from build123d import *
from build123d.topology import SkipClean

# Parameters (mm, degrees)
BOSS_EXTRUDE1_DEPTH     = 12
CUT_EXTRUDE1_DEPTH      = 35.61106579391691
CUT_EXTRUDE1_DEPTH_BACK = 35.61106579391691
BOSS_EXTRUDE2_DEPTH     = 8
CUT_EXTRUDE2_DEPTH      = 2.5
CUT_EXTRUDE3_DEPTH      = 5
SKETCH8_R               = 1.4999999999999996
BOSS_EXTRUDE3_DEPTH     = 5.499999999999998
CUT_EXTRUDE4_DEPTH      = 35.61106579391691
CUT_EXTRUDE4_DEPTH_BACK = 35.61106579391691
SKETCH9_W               = 12
SKETCH9_H               = 6.50766833090351
CUT_EXTRUDE5_DEPTH      = 1


with BuildPart() as part:
    # Sketch1 → Boss-Extrude1 (new body)
    with BuildSketch(Plane.XY):
        with BuildLine():
            Line((-56.57427779976257, 0), (-40.57427779976257, 0))
            Line((-40.57427779976257, 0), (-42.06660946885906, 24.955419174788705))
            ThreePointArc((-42.06660946885906, 24.955419174788705), (-48.57427779976256, 31.463087505692204), (-55.08194613066607, 24.955419174788705))
            Line((-55.08194613066607, 24.955419174788705), (-56.57427779976257, 0))
        make_face()
    extrude(amount=BOSS_EXTRUDE1_DEPTH)

    # Sketch3 → Cut-Extrude1 (cut, two sides: drawn at the far end of the back side and taken through both)
    with BuildSketch(Plane(origin=(-48.57427779976257, 0, 0), x_dir=(0, 0, -1), z_dir=(1, 0, 0)).offset(-CUT_EXTRUDE1_DEPTH_BACK)):
        Polygon((-12, 6.613954943904592), (-12, 0), (-4, -4.9e-16), align=None)
    extrude(amount=CUT_EXTRUDE1_DEPTH + CUT_EXTRUDE1_DEPTH_BACK, mode=Mode.SUBTRACT)

    # Sketch6 → Boss-Extrude2 (add, symmetric)
    with BuildSketch(Plane(origin=(-48.57427779976257, 0, 0), x_dir=(0, 0, -1), z_dir=(1, 0, 0))):
        with BuildLine():
            ThreePointArc((-2.9999999999999982, -1.1000000000000008), (-3.0526985696936526, -0.5401658469562882), (-3.2089428526094457, 4.952e-14))
            Line((-3.2089428526094603, 0), (-4.98019609728148, 0))
            ThreePointArc((-4.980196097281471, 2.665e-14), (-4.62528078247269, -0.499877451714149), (-4.499999999999998, -1.1000000000000008))
            ThreePointArc((-4.499999999999998, -1.1000000000000012), (-6.600122548285821, -2.474719217527322), (-7.0198039027185715, -1.621e-14))
            Line((-7.019803902718577, 0), (-8.7910571473906, 0))
            ThreePointArc((-8.791057147390587, -4.152e-14), (-6.5598341530436635, -4.047301430306355), (-2.9999999999999982, -1.1000000000000014))
        make_face()
        with BuildLine():
            Line((-4.98019609728148, 0), (-3.2089428526094603, 0))
            ThreePointArc((-3.2089428526094457, 4.952e-14), (-6.000000000000047, 1.8999999999999992), (-8.791057147390587, -4.152e-14))
            Line((-8.7910571473906, 0), (-7.019803902718577, 0))
            ThreePointArc((-7.0198039027185715, -1.621e-14), (-6.00000000000003, 0.3999999999999988), (-4.980196097281471, 2.665e-14))
        make_face()
        with BuildLine():
            ThreePointArc((-2.9999999999999982, -1.1000000000000008), (-3.0526985696936526, -0.5401658469562882), (-3.2089428526094457, 4.952e-14))
            Line((-3.2089428526094603, 0), (-4.98019609728148, 0))
            ThreePointArc((-4.980196097281471, 2.665e-14), (-4.62528078247269, -0.499877451714149), (-4.499999999999998, -1.1000000000000008))
            ThreePointArc((-4.499999999999998, -1.1000000000000012), (-6.600122548285821, -2.474719217527322), (-7.0198039027185715, -1.621e-14))
            Line((-7.019803902718577, 0), (-8.7910571473906, 0))
            ThreePointArc((-8.791057147390587, -4.152e-14), (-6.5598341530436635, -4.047301430306355), (-2.9999999999999982, -1.1000000000000014))
        make_face()
        with BuildLine():
            Line((-4.98019609728148, 0), (-3.2089428526094603, 0))
            ThreePointArc((-3.2089428526094457, 4.952e-14), (-6.000000000000047, 1.8999999999999992), (-8.791057147390587, -4.152e-14))
            Line((-8.7910571473906, 0), (-7.019803902718577, 0))
            ThreePointArc((-7.0198039027185715, -1.621e-14), (-6.00000000000003, 0.3999999999999988), (-4.980196097281471, 2.665e-14))
        make_face()
    extrude(amount=BOSS_EXTRUDE2_DEPTH, both=True)

    # Sketch6_3 → Cut-Extrude2 (cut, symmetric)
    with SkipClean():  # the faces are left unmerged after this step: merging them gives an invalid solid
        with BuildSketch(Plane(origin=(-48.57427779976257, 0, 0), x_dir=(0, 0, -1), z_dir=(1, 0, 0))):
            with BuildLine():
                ThreePointArc((-2.9999999999999982, -1.1000000000000008), (-3.0526985696936526, -0.5401658469562882), (-3.2089428526094457, 4.952e-14))
                Line((-3.2089428526094603, 0), (-4.98019609728148, 0))
                ThreePointArc((-4.980196097281471, 2.665e-14), (-4.62528078247269, -0.499877451714149), (-4.499999999999998, -1.1000000000000008))
                ThreePointArc((-4.499999999999998, -1.1000000000000012), (-6.600122548285821, -2.474719217527322), (-7.0198039027185715, -1.621e-14))
                Line((-7.019803902718577, 0), (-8.7910571473906, 0))
                ThreePointArc((-8.791057147390587, -4.152e-14), (-6.5598341530436635, -4.047301430306355), (-2.9999999999999982, -1.1000000000000014))
            make_face()
            with BuildLine():
                Line((-4.98019609728148, 0), (-3.2089428526094603, 0))
                ThreePointArc((-3.2089428526094457, 4.952e-14), (-6.000000000000047, 1.8999999999999992), (-8.791057147390587, -4.152e-14))
                Line((-8.7910571473906, 0), (-7.019803902718577, 0))
                ThreePointArc((-7.0198039027185715, -1.621e-14), (-6.00000000000003, 0.3999999999999988), (-4.980196097281471, 2.665e-14))
            make_face()
            with BuildLine():
                ThreePointArc((-2.9999999999999982, -1.1000000000000008), (-3.0526985696936526, -0.5401658469562882), (-3.2089428526094457, 4.952e-14))
                Line((-3.2089428526094603, 0), (-4.98019609728148, 0))
                ThreePointArc((-4.980196097281471, 2.665e-14), (-4.62528078247269, -0.499877451714149), (-4.499999999999998, -1.1000000000000008))
                ThreePointArc((-4.499999999999998, -1.1000000000000012), (-6.600122548285821, -2.474719217527322), (-7.0198039027185715, -1.621e-14))
                Line((-7.019803902718577, 0), (-8.7910571473906, 0))
                ThreePointArc((-8.791057147390587, -4.152e-14), (-6.5598341530436635, -4.047301430306355), (-2.9999999999999982, -1.1000000000000014))
            make_face()
            with BuildLine():
                Line((-4.98019609728148, 0), (-3.2089428526094603, 0))
                ThreePointArc((-3.2089428526094457, 4.952e-14), (-6.000000000000047, 1.8999999999999992), (-8.791057147390587, -4.152e-14))
                Line((-8.7910571473906, 0), (-7.019803902718577, 0))
                ThreePointArc((-7.0198039027185715, -1.621e-14), (-6.00000000000003, 0.3999999999999988), (-4.980196097281471, 2.665e-14))
            make_face()
        extrude(amount=CUT_EXTRUDE2_DEPTH, both=True, mode=Mode.SUBTRACT)

    # Sketch7 → Cut-Extrude3 (cut, symmetric)
    with SkipClean():  # the faces are left unmerged after this step: merging them gives an invalid solid
        with BuildSketch(Plane(origin=(-48.57427779976257, 0, 0), x_dir=(0, 0, -1), z_dir=(1, 0, 0))):
            Polygon((-7.161655697006073, 2.6138810410171796), (-11.015220244212237, 5.799793827098392), (-7.829307458131025, 9.653358374304556), (-3.9757429109248625, 6.467445588223342), align=None)
        extrude(amount=CUT_EXTRUDE3_DEPTH, both=True, mode=Mode.SUBTRACT)

    # Sketch8 → Boss-Extrude3 (add, symmetric)
    with SkipClean():  # the faces are left unmerged after this step: merging them gives an invalid solid
        with BuildSketch(Plane(origin=(-48.57427779976257, 0, 0), x_dir=(0, 0, -1), z_dir=(1, 0, 0))):
            with Locations((-7.548090255966457, 6.177113636233633)):
                Circle(SKETCH8_R)
        extrude(amount=BOSS_EXTRUDE3_DEPTH, both=True)

    # Sketch9 → Cut-Extrude4 (cut, two sides: drawn at the far end of the back side and taken through both)
    with SkipClean():  # the faces are left unmerged after this step: merging them gives an invalid solid
        with BuildSketch(Plane(origin=(-48.57427779976257, 0, 0), x_dir=(0, 0, -1), z_dir=(1, 0, 0)).offset(-CUT_EXTRUDE4_DEPTH_BACK)):
            with Locations((-6, 28.20925334024046)):
                Rectangle(SKETCH9_W, SKETCH9_H)
        extrude(amount=CUT_EXTRUDE4_DEPTH + CUT_EXTRUDE4_DEPTH_BACK, mode=Mode.SUBTRACT)

    # Sketch10 → Cut-Extrude5 (cut, symmetric)
    with SkipClean():  # the faces are left unmerged after this step: merging them gives an invalid solid
        with BuildSketch(Plane(origin=(-48.57427779976257, 0, 0), x_dir=(0, 0, -1), z_dir=(1, 0, 0))):
            Polygon((-2.32, -2.8e-16), (-0.31999999999999995, -2e-17), (-0.31999999999999995, 0.8014860865112553), (-0.31999999999999995, 27.37726434659022), (-2.32, 27.37726434659022), (-2.32, 0.8014860865112539), align=None)
        extrude(amount=CUT_EXTRUDE5_DEPTH, both=True, mode=Mode.SUBTRACT)


solid = part.part
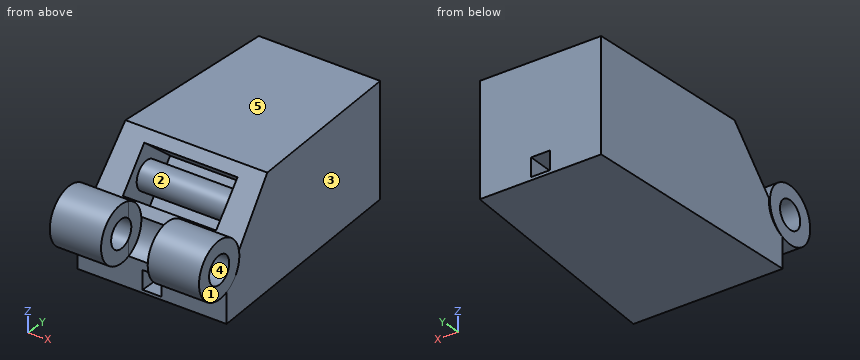
The listing builds one solid part. Answer for the finished solid, in the listing's coordinates (mm). Face numbers are marked on the shaded views. A direction names the side the tool comes from. Give positions to 0.01 mm unless a question says otherwise; leave off trailing zeros. Write each loop counter-clockwise with the first axis right and the second up, starting at its lowest first coordinate (ties: lowest second). Pieces come first, ordered by that corner, then holes.
Item 1: Flat-ended cylindrical pins translate along their axes: P1, Ø1.5, axis at x = -48, y = 1.5, coming from the +Z side; P2, Ø4, axis at y = 13.5, z = 7, coming from the +X side; P3, Ø1.8, axis at y = -1.1, z = 6, coming from the -X side; P4, Ø1, axis at x = -49, z = 9, coming from the -Y side. Find the tip coordinate at first contact, or state that the pin passes through.
Item 2: Section C-C, the plane y = -1.1 is taken. Write down the section's boundary in (x, z), plus the area to 3 significant figures.
Item 3: Determine the mould class of the marked faces 3, 4 and 5 for opening direction Z: released by +Z, released by -Z, zero draft, split by the parting line, or undercut.
Item 4: Which of the six approach directions +Z, -Z, +X, -X, +Y, -Y give full straight-line access (tool end or side, diameter ignored) to the marked faces 1 and 2?
Item 5: Find the intervals of material crossed by line 1 along Z through (x, y) = (-43.4, -1.1); line 2 along X through (y, z) = (-0.5, 4.25); line 3 along Y through (x, z) = (-54.3, 6), in increasing order.
Item 6: Section A-A, the plane z = 1.75 is taken. Write down the section's boundary in (x, y).
Item 7: Section D-D, the plane y = 8.75 is taken. Write down the section's boundary in (x, z), plus the area to 3 significant figures.
Item 8: Section B-B, the plane x = -45.75 is taken. Write down the section's boundary in (y, z), plus the area to 3 significant figures.
Completed:
1. P1: stops at z = 6.72
1. P2: stops at x = -41.26
1. P3: passes through
1. P4: stops at y = 5.02
2. outline: (-56.57, 3) - (-51.07, 3) - (-51.07, 4.5) - (-56.57, 4.5) - close; (-56.57, 7.5) - (-51.07, 7.5) - (-51.07, 9) - (-56.57, 9) - close; (-46.07, 3) - (-40.57, 3) - (-40.57, 4.5) - (-46.07, 4.5) - close; (-46.07, 7.5) - (-40.57, 7.5) - (-40.57, 9) - (-46.07, 9) - close
2. area: 33.0 mm2
3. face 3: zero draft
3. face 4: undercut
3. face 5: released by +Z
4. face 1: +Z, -Z, +X, +Y, -Y
4. face 2: none
5. line 1: z = 3 to 4.5, 7.5 to 9
5. line 2: x = -56.57 to -51.07, -46.07 to -40.57
5. line 3: y = -4.1 to -2.6, 0.4 to 24.96
6. outline: (-56.57, 0) - (-49.57, 0) - (-49.57, 24.96) - (-55.08, 24.96) - close; (-47.57, 0) - (-40.57, 0) - (-42.07, 24.96) - (-47.57, 24.96) - close
7. outline: (-56.05, 0) - (-41.1, 0) - (-41.1, 12) - (-56.05, 12) - close; hole (-53.57, 6.74) - (-43.57, 6.74) - (-43.57, 8.58) - (-53.57, 8.58) - close; hole (-49.57, 0.32) - (-47.57, 0.32) - (-47.57, 2.32) - (-49.57, 2.32) - close
7. area: 157 mm2
8. outline: (0, 0) - (24.96, 0) - (24.96, 12) - (6.61, 12) - (5.8, 11.02) - (9.65, 7.83) - (6.47, 3.98) - (2.61, 7.16) - (1.89, 6.28) arc R3 ccw (long way) to (0, 3.21) - close; circle Ø3 at (6.18, 7.55); hole circle Ø3 at (-1.1, 6)
8. area: 274 mm2
